```python
from build123d import *

# Parameters (mm, degrees)
SKETCH016_R  = 3
PAD017_DEPTH = 20
SKETCH020_W  = 2.5
SKETCH020_H  = 16.93
PAD021_DEPTH = 18


with BuildPart() as obj1:
    # Sketch016 → Pad017 (new body)
    with BuildSketch(Plane.XY):
        with BuildLine():
            ThreePointArc((-121.92, -35.56), (-116.758725, -45.780451), (-105.46998, -47.693728))
            Line((-105.46998, -46.223728), (-105.46998, -47.693728))
            Line((-111.96998, -46.223728), (-105.46998, -46.223728))
            Line((-111.96998, -43.123728), (-111.96998, -46.223728))
            Line((-105.46998, -43.123728), (-111.96998, -43.123728))
            Line((-105.46998, -31.693728), (-105.46998, -43.123728))
            Line((-105.46998, -31.693728), (-105.46998, -26.193728))
            ThreePointArc((-105.46998, -26.193728), (-105.669987, -25.66457), (-106.17, -25.4))
            Line((-106.17, -25.4), (-121.92, -25.4))
            Line((-121.92, -25.4), (-121.92, -35.56))
        make_face()
        with Locations((-109.22, -35.56)):
            Circle(SKETCH016_R, mode=Mode.SUBTRACT)
    extrude(amount=PAD017_DEPTH)

    # Sketch020 (on Face13 of Pad017) → Pad021 (join)
    with BuildSketch(Plane.XY.offset(20)):
        with Locations((-104.21998, -34.658728)):
            Rectangle(SKETCH020_W, SKETCH020_H)
    extrude(amount=-PAD021_DEPTH)


with BuildPart() as obj1_1:
    # Body012 placement: moved
    add(obj1.part.moved(Location((0, 19, 0))))


with BuildPart() as obj1_mirrored:
    # mirror: instance of obj1
    add(obj1_1.part.mirror(Plane(origin=(0, 0, 0), x_dir=(0, -1, 0), z_dir=(1, 0, 0))))


solid = obj1_mirrored.part
```
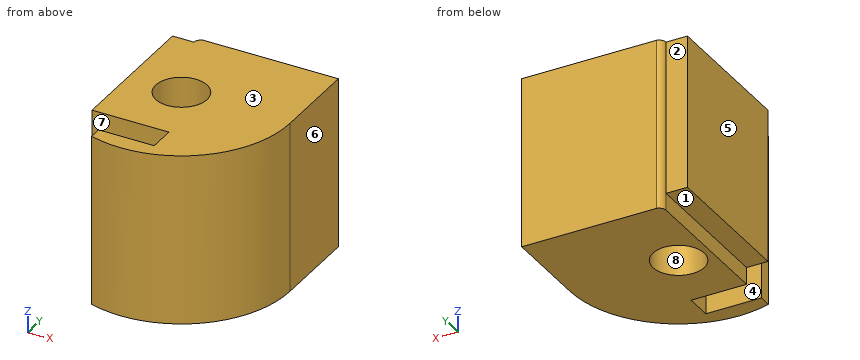
For this review, take the finished solid that the model builds, in its own axes (mm). Face numbers are marked on the shaded views. A direction names the side the tool comes from. Round coordinates to 2 decimals unless told otherwise and drop trailing zeros. Write each loop counter-clockwise with the first axis right and the second up, starting at its lowest first coordinate (ties: lowest second). Pieces come first, ordered by that corner, then holes. Notation, with made-up numbers: (62, 44.25) -> (79, 44.25) arc R27 cw to (79, 68.25) -> close; hole circle Ø4 at (-37, -34.75). An arc over 180 degrees is marked (long way). One line per question, with ' | ' between items. Start each with the question number.
(1) Tool access review of the marked faces 1, 2, 3, 4 and 5: name each direction out of +Z, -Z, +X, -X, +Y, -Y from which nothing blocks a thin tool from reaching the whole face with its end or side.
(2) For line 1 along Y through (x, z) = (109.22, 8.5); line 2 along Y through (x, z) = (111.5, 4); line 3 along Y through (x, z) = (105.25, 3.5), list the stretches that pass through material, from the lowest coordinate up. Write a range as from..to.
(3) Mouldability with a two-part tool opening along X and no side actions: class the marked faces 6, 7 and 8 as released by +X, released by -X, zero draft, split by the parting line, or undercut.
(4) Insertion check: P1, Ø0.6, axis at y = -12, z = 1.5, coming from the -X side. The pin has a flat end and moves straight along its axis. Give the tip position at first contact, or say it passes through.
(5) Add section D-D, the plane y = -21.25. Write out the cut boundary in (x, z).
(6) Add section C-C, the plane y = -18.5. Write out the cut boundary in (x, z).
(7) Add section A-A, the plane x = 109.22. Write out the cut boundary in (y, z).
(8) Add section B-B, the plane z = 3.5. Write out the cut boundary in (x, y), plus the area to 4 significant figures.
Answer list:
1) face 1: -Z, -X, +Y, -Y | face 2: +Z, -Z, -X, +Y | face 3: +Z, +X, -X, +Y, -Y | face 4: +Z, -Z, -X | face 5: +Z, -Z, -X, +Y, -Y
2) line 1: -29.26..-27.22, -24.12..-19.56, -13.56..-6.4 | line 2: -29.05..-27.22, -24.12..-18.51, -14.61..-6.4 | line 3: -24.12..-7.19
3) face 6: released by +X | face 7: zero draft | face 8: undercut
4) P1: x = 105.47
5) outline: (102.97, 2) -> (105.47, 2) -> (105.47, 0) -> (121.02, 0) -> (121.02, 20) -> (102.97, 20) -> close
6) outline: (102.97, 2) -> (105.47, 2) -> (105.47, 0) -> (106.93, 0) -> (106.93, 20) -> (102.97, 20) -> close; (111.51, 0) -> (121.77, 0) -> (121.77, 20) -> (111.51, 20) -> close
7) outline: (-29.26, 0) -> (-27.22, 0) -> (-27.22, 20) -> (-29.26, 20) -> close; (-24.12, 0) -> (-19.56, 0) -> (-19.56, 20) -> (-24.12, 20) -> close; (-13.56, 0) -> (-6.4, 0) -> (-6.4, 20) -> (-13.56, 20) -> close
8) outline: (102.97, -24.12) -> (111.97, -24.12) -> (111.97, -27.22) -> (105.47, -27.22) -> (105.47, -28.69) arc R12.7 ccw to (121.92, -16.56) -> (121.92, -6.4) -> (106.17, -6.4) arc R0.8 ccw to (105.47, -7.19) -> (102.97, -7.19) -> close; hole circle Ø6 at (109.22, -16.56) | area: 334.5 mm²
